Source: CAD feature listing. Evaluate the final solid. Frame: model axes, mm. Face numbers are marked on the shaded views. A direction names the side the tool comes from. Coordinates: 2 decimals unless noted, no trailing zeros. Loops run counter-clockwise (first coordinate to the right, second up) from the corner with the lowest first, then second, coordinate; pieces in that order, holes last. Notation, with made-up numbers: (43, 41.25) - (99, 41.25) arc R30 ccw to (99, 73.25) - close; hole circle Ø4 at (66.5, 18). An arc over 180 degrees is marked (long way). Use CSV: the item, a comma, the result in double quotes. Start each with the question number.
```python
from build123d import *

# Parameters (mm, degrees)
SKETCH2_R           = 19.05
SKETCH3_R           = 33.02
BOSS_EXTRUDE1_DEPTH = 19.05
SKETCH4_W           = 12.7
SKETCH4_H           = 14.313474639


with BuildPart() as part:
    # Sweep1: sweep along a path in Sketch1
    with BuildLine(Plane.XY) as sweep1_path:
        Line((0, 82.55), (0, 0))
        Line((0, 0), (127, 0))
    # Sketch2 → Sweep1 (sweep)
    with BuildSketch(Plane(origin=(127, 0, 0), x_dir=(0, 0, -1), z_dir=(1, 0, 0))):
        Circle(SKETCH2_R)
    sweep(path=sweep1_path.line, transition=Transition.RIGHT)

    # Sketch3 → Boss-Extrude1 (add)
    with BuildSketch(Plane(origin=(0, 82.55, 0), x_dir=(1, 0, 0), z_dir=(0, 1, 0))):
        with Locations(Location((0, 0, 0), (0, 0, 180))):
            Circle(SKETCH3_R)
    extrude(amount=-BOSS_EXTRUDE1_DEPTH)

    # Sketch4 → Revolve1 (revolve)
    with BuildSketch(Plane.XY, mode=Mode.PRIVATE) as revolve1_sk:
        with Locations((120.65, 26.20673732)):
            Rectangle(SKETCH4_W, SKETCH4_H)
        with Locations((57.15, 26.20673732)):
            Rectangle(SKETCH4_W, SKETCH4_H)
    revolve(revolve1_sk.sketch.rotate(Axis((0, 0, 0), (1, 0, 0)), 90), axis=Axis((0, 0, 0), (1, 0, 0)))


solid = part.part
```
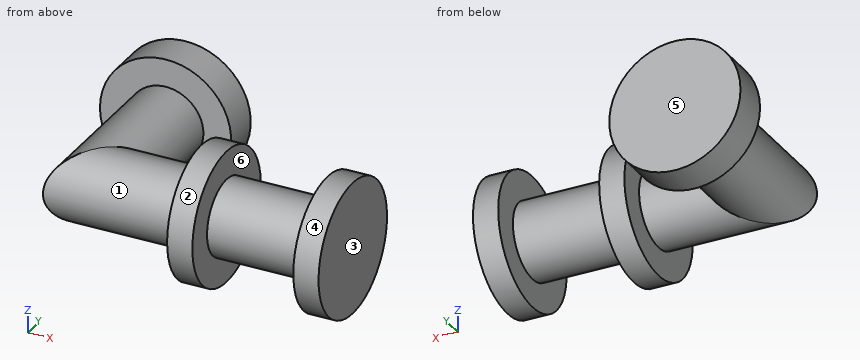
(1) Section D-D on z = 0. Output: boundary loops of the cut face in (x, y).
(2) Draft query along Y for the marked faces 1, 2 and 3. Return one class per face: released by +Y, released by -Y, zero draft, split by the parting line, or undercut.
(3) Reachability of the marked faces 4, 5 and 6 from +Z, -Z, +X, -X, +Y, -Y: full face, straight path, thin tool, end or side. Return the list, or none.
(4) Ray query, line 1 (X direction, y = 14, z = -29); line 2 (Y direction, x = 34, z = -0.5); line 3 (Y direction, x = 4, z = 22). Return the intervals inside material, ascending. Write a range as [from, to].
(5) Section B-B on z = 25. Output: boundary loops of the cut face in (x, y), plus the area to 3 significant figures.
(6) Section C-C on x = 0. Output: boundary loops of the cut face in (y, z).
(7) Pin query (flat end, axial travel): pin 1 Ø12 at (x, y) = (48.5, 13) entering from +Z; pin 2 Ø5 at (x, z) = (29, 23.5) entering from +Y; pin 3 Ø20 at (x, z) = (-10, -3) entering from -Y; pin 4 Ø12 at (y, z) = (44, -3) entering from -X. Return the tip coordinate at first contact, or that it passes through.
(8) Section A-A on y = 25. Output: boundary loops of the cut face in (x, z), plus the area to 3 significant figures.
Solution:
1,outline,"(-33.02, 63.5) - (-19.05, 63.5) - (-19.05, -19.05) - (50.8, -19.05) - (50.8, -33.36) - (63.5, -33.36) - (63.5, -19.05) - (114.3, -19.05) - (114.3, -33.36) - (127, -33.36) - (127, 33.36) - (114.3, 33.36) - (114.3, 19.05) - (63.5, 19.05) - (63.5, 33.36) - (50.8, 33.36) - (50.8, 19.05) - (19.05, 19.05) - (19.05, 63.5) - (33.02, 63.5) - (33.02, 82.55) - (-33.02, 82.55) - close"
2,face 1,"undercut"
2,face 2,"split by the parting line"
2,face 3,"zero draft"
3,face 4,"+X"
3,face 5,"+Z, -Z, +X, -X, +Y"
3,face 6,"none"
4,line 1,"x = [50.8, 63.5], [114.3, 127]"
4,line 2,"y = [-19.04, 19.04]"
4,line 3,"y = [63.5, 82.55]"
5,outline,"(-21.57, 63.5) - (21.57, 63.5) - (21.57, 82.55) - (-21.57, 82.55) - close; (50.8, -22.09) - (63.5, -22.09) - (63.5, 22.09) - (50.8, 22.09) - close; (114.3, -22.09) - (127, -22.09) - (127, 22.09) - (114.3, 22.09) - close"
5,area,"1,940 mm²"
6,outline,"(0, -19.05) - (63.5, -19.05) - (63.5, -33.02) - (82.55, -33.02) - (82.55, 33.02) - (63.5, 33.02) - (63.5, 19.05) - (0, 19.05) arc R19.05 ccw to start"
7,pin 1,"stops at z = 32.52"
7,pin 2,"passes through"
7,pin 3,"stops at y = -19.05"
7,pin 4,"stops at x = -19.05"
8,outline,"circle Ø38.1 at (0, 0); (50.8, -22.09) - (63.5, -22.09) - (63.5, 22.09) - (50.8, 22.09) - close; (114.3, -22.09) - (127, -22.09) - (127, 22.09) - (114.3, 22.09) - close"
8,area,"2,260 mm²"
